Verification items for the finished model (mm, model axes). Round coordinates to 2 decimals unless told otherwise and drop trailing zeros. Order: outer loops, then holes, each group sorted by start corner. A loop starts at its lowest first (then second) coordinate and runs counter-clockwise, first axis right, second up. Notation, with made-up numbers: (-39, -23.5) -> (11, -23.5) arc R35 cw to (11, 13.5) -> close; hole circle Ø2 at (61.25, -21). An arc over 180 degrees is marked (long way). Return JSON: item names as keys, results as strings. Group by question number.
1) Section check A-A on x = -2.5. Enter the section's corners in (y, z).
2) Depth check by flat-ended pin: pin 1 (16.5 mm diameter, centred on x = 5, z = -95, fed in from -Y); pin 2 (1.8 mm diameter, centred on x = -9, y = 3.5, fed in from +Z); pin 3 (0.7 mm diameter, centred on x = -9, y = 1.5, fed in from -Z). Enter the tip coordinate at first touch or a pass-through.
3) Section check B-B on y = 3. Enter the section's corners in (x, z), plus the area to 3 significant figures.
4) Scan lines: L1, parallel to Z at x = -16, y = 0.6; L2, parallel to Z at x = -4, y = 2.7; L3, parallel to Y at x = 9.5, z = -88.5. Record each from-to range of solid material in increasing order.
```python
from build123d import *

# Parameters (mm, degrees)
SKETCH_1_W          = 38.8
SKETCH_1_H          = 200
EXTRUDE_1_DEPTH     = 4.4
SKETCH_2_W          = 38.8
SKETCH_2_H          = 15
CUT_EXTRUDE_1_DEPTH = 2.2
SKETCH_3_W          = 38.8
SKETCH_3_H          = 15
CUT_EXTRUDE_2_DEPTH = 2.2


with BuildPart() as part:
    # 草圖1 → 填料-伸長1 (new body)
    with BuildSketch(Plane(origin=(0, 0, 0), x_dir=(1, 0, 0), z_dir=(0, 1, 0))):
        Rectangle(SKETCH_1_W, SKETCH_1_H)
    extrude(amount=EXTRUDE_1_DEPTH)

    # 草圖2 → 除料-伸長1 (cut)
    with BuildSketch(Plane(origin=(0, 4.4, 0), x_dir=(1, 0, 0), z_dir=(0, 1, 0))):
        with Locations((0, -92.5)):
            Rectangle(SKETCH_2_W, SKETCH_2_H)
    extrude(amount=-CUT_EXTRUDE_1_DEPTH, mode=Mode.SUBTRACT)

    # 草圖3 → 除料-伸長2 (cut)
    with BuildSketch(Plane.XZ):
        with Locations((0, -92.5)):
            Rectangle(SKETCH_3_W, SKETCH_3_H)
    extrude(amount=-CUT_EXTRUDE_2_DEPTH, mode=Mode.SUBTRACT)


solid = part.part
```
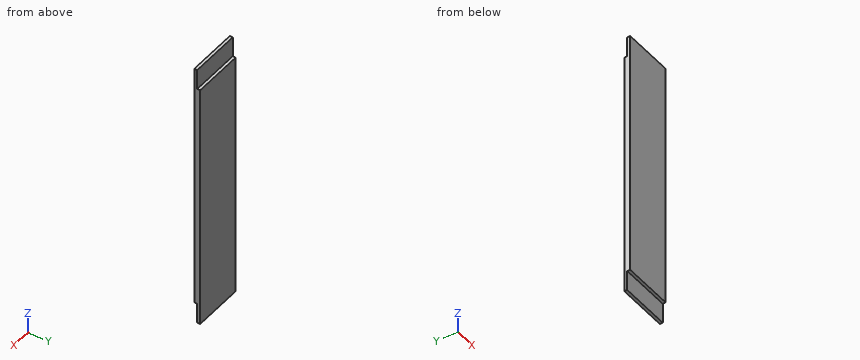
Check result:
{
 "1": {"outline": "(0, -85) -> (2.2, -85) -> (2.2, -100) -> (4.4, -100) -> (4.4, 85) -> (2.2, 85) -> (2.2, 100) -> (0, 100) -> close"},
 "2": {"pin 1": "y = 2.2", "pin 2": "z = 85", "pin 3": "z = -85"},
 "3": {"outline": "(-19.4, -100) -> (19.4, -100) -> (19.4, 85) -> (-19.4, 85) -> close", "area": "7,180 mm^2"},
 "4": {"L1": "-85 to 100", "L2": "-100 to 85", "L3": "2.2 to 4.4"}
}
